Here's how the part is built. I have some questions about the finished solid (model axes, mm). Face numbers are marked on the shaded views. A direction names the side the tool comes from. Coordinates: 2 decimals unless noted, no trailing zeros. Write each loop counter-clockwise with the first axis right and the second up, starting at its lowest first coordinate (ties: lowest second). Pieces come first, ordered by that corner, then holes.
Item 1: I'm going to push flat-ended pins straight in: P1, Ø1.8, axis at y = -7, z = -7, coming from the -X side; P2, Ø5, axis at x = 29.8, z = 9, coming from the +Y side; P3, Ø9.5, axis at x = 14, y = -3.5, coming from the +Z side; P4, Ø1.5, axis at y = 0, z = 8, coming from the -X side. Where does each tip first touch, or does it pass through?
Item 2: If we mould it in two halves opening along Z, with no side actions, what happens to the marked faces 1, 2 and 3? For each: pulls with the +Z half, pulls with the -Z half, needs draft (parallel to the pull), parting line crosses it, or undercut.
Item 3: I want a section at D-D (y = 2.25). Please give me the cut outline in (x, z).
Item 4: Please list where these lines run through material, in increasing order: line 1 (Y direction, x = 2.25, z = -7); line 2 (Y direction, x = 24, z = -6); line 3 (X direction, y = -0.7, z = 9).
Item 5: I want a section at A-A (x = 47.2). Please give me the cut outline in (y, z), and give its area (3 significant figures).
Item 6: For the marked faces 4, 5, 6 and 7, which set-ups out of +Z, -Z, +X, -X, +Y, -Y let a thin tool reach every point of the face, with its end or its side?
Item 7: I want a section at C-C (x = 3). Please give me the cut outline in (y, z).
Item 8: I want a section at B-B (y = -7). Please give me the cut outline in (x, z).
from build123d import *

# Parameters (mm, degrees)
SKETCH_1_R      = 1.5
EXTRUDE_1_DEPTH = 3
SKETCH_2_W      = 14
SKETCH_2_H      = 20
SKETCH_2_R      = 1.5
EXTRUDE_2_DEPTH = 6
CHAMFER_1_SIZE  = 2
CHAMFER_2_SIZE  = 6
CHAMFER_3_SIZE  = 5


with BuildPart() as part:
    # 草图1 → 凸台-拉伸1 (new, symmetric)
    with BuildSketch(Plane(origin=(0, 0, 0), x_dir=(1, 0, 0), z_dir=(0, 1, 0))):
        Polygon((0, 14), (0, 0), (25, 0), (25, -14), (55, -14), (55, 14), align=None)
        with Locations(Location((25, 9, 0), (0, 0, 270))):
            Circle(SKETCH_1_R, mode=Mode.SUBTRACT)
        with Locations(Location((52, 1, 0), (0, 0, 270))):
            Circle(SKETCH_1_R, mode=Mode.SUBTRACT)
        with Locations(Location((29.8, -9, 0), (0, 0, 270))):
            Circle(SKETCH_1_R, mode=Mode.SUBTRACT)
        with Locations(Location((47.2, -1, 0), (0, 0, 270))):
            Circle(SKETCH_1_R, mode=Mode.SUBTRACT)
    extrude(amount=EXTRUDE_1_DEPTH, both=True)

    # 草图2 → 凸台-拉伸2 (add)
    with BuildSketch(Plane(origin=(0, 0, 0), x_dir=(0, 0, -1), z_dir=(1, 0, 0))):
        with Locations((7, 0)):
            Rectangle(SKETCH_2_W, SKETCH_2_H)
        with Locations((7, 7)):
            Circle(SKETCH_2_R, mode=Mode.SUBTRACT)
        with Locations((7, -7)):
            Circle(SKETCH_2_R, mode=Mode.SUBTRACT)
    extrude(amount=EXTRUDE_2_DEPTH)

    # 倒角1
    # the kernel refuses this chamfer: 2 mm, written as the material it takes off along each edge
    with BuildSketch(Plane(origin=(6, 7, -7), x_dir=(0, 0, -1), z_dir=(0, -1, 0))) as chamfer_1_piece_1:
        Polygon((1.5, -CHAMFER_1_SIZE), (1.5 + CHAMFER_1_SIZE, 0), (1.5, 0), align=None)
    revolve(axis=Axis((6, 7, -7), (1, 0, 0)), mode=Mode.SUBTRACT)
    with BuildSketch(Plane(origin=(6, -7, -7), x_dir=(0, 0, -1), z_dir=(0, -1, 0))) as chamfer_1_piece_2:
        Polygon((1.5 + CHAMFER_1_SIZE, 0), (1.5, -CHAMFER_1_SIZE), (1.5, 0), align=None)
    revolve(axis=Axis((6, -7, -7), (1, 0, 0)), mode=Mode.SUBTRACT)

    # 倒角2
    chamfer_2_edges = [part.edges().sort_by_distance(p)[0] for p in [
        (25, 0, 0),
    ]]
    chamfer(chamfer_2_edges, length=CHAMFER_2_SIZE)

    # 倒角3
    chamfer_3_edges = [part.edges().sort_by_distance(p)[0] for p in [
        (55, 0, -14),
        (55, 0, 14),
        (25, 0, 14),
    ]]
    chamfer(chamfer_3_edges, length=CHAMFER_3_SIZE)


solid = part.part
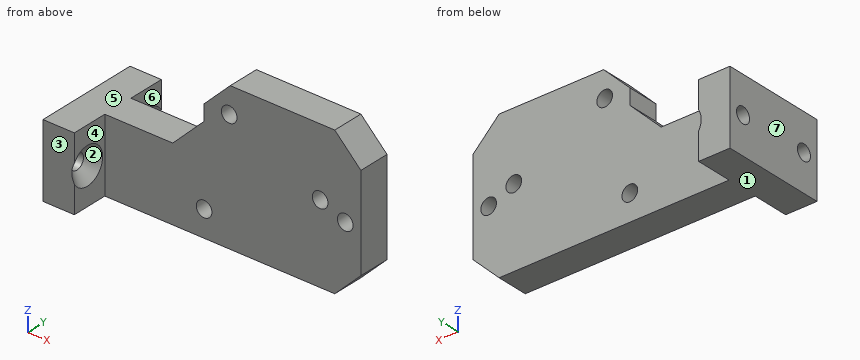
Answer:
1. P1: passes through
1. P2: stops at y = 3
1. P3: stops at z = 0
1. P4: stops at x = 25
2. face 1: pulls with the -Z half
2. face 2: undercut
2. face 3: needs draft
3. outline: (0, -14) - (50, -14) - (55, -9) - (55, 9) - (50, 14) - (30, 14) - (25, 9) - (25, 6) - (19, 0) - (0, 0) - close; hole circle Ø3 at (25, -9); hole circle Ø3 at (29.8, 9); hole circle Ø3 at (47.2, 1); hole circle Ø3 at (52, -1)
4. line 1: y = -10 to -8.5, -5.5 to 5.5, 8.5 to 10
4. line 2: y = -3 to 3
4. line 3: x = 25 to 28.3, 31.3 to 55
5. outline: (-3, -14) - (3, -14) - (3, -0.5) - (-3, -0.5) - close; (-3, 2.5) - (3, 2.5) - (3, 14) - (-3, 14) - close
5. area: 150 mm2
6. face 4: +Z, -Z, +X, -Y
6. face 5: +Z, -X, +Y, -Y
6. face 6: +Z, -Z, +X, +Y
6. face 7: +Z, -Z, -X, +Y, -Y
7. outline: (-10, -14) - (10, -14) - (10, 0) - (-10, 0) - close; hole circle Ø3 at (-7, -7); hole circle Ø3 at (7, -7)
8. outline: (0, -14) - (6, -14) - (6, -10.5) - (4, -8.5) - (0, -8.5) - close; (0, -5.5) - (4, -5.5) - (6, -3.5) - (6, 0) - (0, 0) - close
